Autodesk Inventor part; units mm, degrees
ref_plane "YZ Plane" through (0, 0, 0) normal (1, 0, 0) x (0, 1, 0)
ref_plane "XZ Plane" through (0, 0, 0) normal (0, 1, 0) x (-1, 0, 0)
ref_plane "XY Plane" through (0, 0, 0) normal (0, 0, 1) x (1, 0, 0)
sketch "Эскиз1" plane through (0, 0, 0) normal (0, 1, 0) x (-1, 0, 0)
  line L0 (-150, 85) -> (150, 85)
  line L1 (150, 85) -> (150, -85)
  line L2 (150, -85) -> (-150, -85)
  line L3 (-150, -85) -> (-150, 85)
  line L4 (-150, 85) -> (150, -85) construction
  line L5 (150, 85) -> (-150, -85) construction
  point P0 (0, 0)
  dimension "d0" = 170
  dimension "d1" = 300
extrude "Выдавливание1" add sketch "Эскиз1" along normal blind 3
sketch "Эскиз4" plane through (0, 0, 0) normal (0, -1, 0) x (1, 0, 0)
  line L0 (150, -85) -> (-150, -85)
  line L1 (150, 85) -> (150, -85)
  line L2 (-150, 85) -> (150, 85)
  line L3 (-150, -85) -> (-150, 85)
  line L4 (150, -85) -> (-150, -85)
  line L5 (-150, -85) -> (-150, 85)
  line L6 (-150, 85) -> (-78, 85)
  line L7 (-78, 85) -> (-78, -85)
  line L8 (-78, -85) -> (-150, -85)
  point P0 (0, 0)
  point P1 (-78, -85)
  point P2 (-78, 85)
  dimension "d17" = 72
extrude "Выдавливание3" add sketch "Эскиз4" along normal blind 2 contours L0 L3 L2 L7
sketch "Эскиз2" plane through (0, 3, 0) normal (0, 1, 0) x (1, 0, 0)
  line L0 (-82, 81) -> (-146, 81) construction
  line L1 (-146, 81) -> (-146, -81) construction
  line L2 (-146, -81) -> (-82, -81) construction
  line L3 (-82, -81) -> (-82, 81) construction
  line L4 (-82, 81) -> (-146, -81) construction
  line L5 (-146, 81) -> (-82, -81) construction
  line L6 (0, 0) -> (-69.8255, 0) construction
  line L7 (-150, 85) -> (-150, -85) construction
  point P0 (-114, 0)
  point P1 (-114, 0)
  dimension "d4" = 162
  dimension "d5" = 4
  dimension "d6" = 64
hole "Отверстие1" at (-146, 3, 81) at (-82, 3, 81) at (-146, 3, -81) at (-82, 3, -81) direction (0, -1, 0) diameter 3.4 depth 3.7 countersink diameter 6.6 countersink angle 90
fillet "Сопряжение1" radius 0.5 2 edges at (-78, 0, 0) (-78, -2, 0)
properties part number "форточка"
Verification items for the finished model (mm, model axes). A direction names the side the tool comes from. Coordinates: 2 decimals unless noted, no trailing zeros. Order: outer loops, then holes, each group sorted by start corner. A loop starts at its lowest first (then second) coordinate and runs counter-clockwise, first axis right, second up. Notation, with made-up numbers: (36.5, -5.5) -> (88.5, -5.5) arc R17 cw to (88.5, 21.5) -> close; hole circle Ø2 at (68, -31). An arc over 180 degrees is marked (long way). Put each result on its own line as item: value. Start each with the question number.
1. Cross-section at A-A, the plane z = 23. Record the boundary of the cut face in (x, y).
2. Access from +Z, -Z, +X, -X, +Y, -Y to the whole of each face (thin tool, end or side, straight path). Record for faces 1 (the flat face through (38, 0, 1)), 2 (the flat face through (2, 3, 1)).
3. Material ranges on L1, parallel to Z at x = -82, y = 1; L2, parallel to X at y = -0.3, z = 81; L3, parallel to X at y = 0.8, z = 81, recorded low to high. Write a range as [from, to].
4. Go/stop test with flat-tipped pins: pin 1 Ø1.7 at (x, z) = (-81.5, -81.5) entering from +Y; pin 2 Ø4.5 at (x, z) = (-146, -81) entering from +Y; pin 3 Ø5.5 at (x, z) = (-82, 81) entering from +Y. Record where each tip stops, or that it passes through.
5. Cross-section at B-B, the plane x = -68.5. Record the boundary of the cut face in (y, z), then the cut area to 3 significant figures.
Computed:
1. outline: (-150, -2) -> (-78.5, -2) arc R0.5 ccw to (-78, -1.5) -> (-78, -0.5) arc R0.5 cw to (-77.5, 0) -> (150, 0) -> (150, 3) -> (-150, 3) -> close
2. face 1: +Z, -Z, +X, -Y
2. face 2: +Z, -Z, +X, -X, +Y
3. L1: [-85, -82.7], [-79.3, 79.3], [82.7, 85]
3. L2: [-150, -147.7], [-144.3, -83.7], [-80.3, -77.96]
3. L3: [-150, -147.7], [-144.3, -83.7], [-80.3, 150]
4. pin 1: y = -0.7
4. pin 2: y = 1.95
4. pin 3: y = 2.45
5. outline: (0, -85) -> (3, -85) -> (3, 85) -> (0, 85) -> close
5. area: 510 mm2
